Geometry check sheet. Reference: the model listing, model coordinates, mm. Face numbers are marked on the shaded views. A direction names the side the tool comes from. Give positions to 0.01 mm unless a question says otherwise; leave off trailing zeros. Write each loop counter-clockwise with the first axis right and the second up, starting at its lowest first coordinate (ties: lowest second). Pieces come first, ordered by that corner, then holes. Notation, with made-up numbers: (85.5, -34) -> (108.5, -34) arc R8 ccw to (108.5, -27) -> close; hole circle Ø1 at (35.25, 31.5). An arc over 180 degrees is marked (long way). Write item = value, one per line. Start each with the question number.
1. Set-up check for the marked faces 1 and 2: record each of +Z, -Z, +X, -X, +Y, -Y from which the full face is reachable in a straight line by a thin tool's end or side.
2. Thickness scan on line 1 along Y through (x, z) = (9.5, 4). Record the ranges inside material, lowest first.
3. Depth check by flat-ended pin: P1, Ø9.5, axis at y = 8.5, z = 12, coming from the +X side; P2, Ø12, axis at x = 12, y = 11, coming from the +Z side; P3, Ø10, axis at x = 5.5, y = 9, coming from the +Z side. Enter the tip coordinate at first touch or a pass-through.
4. Cross-section at A-A, the plane y = 7.25. Record the cut outline in (x, z).
```python
from build123d import *

# Parameters (mm, degrees)
F1_DEPTH     = 20
F3_DEPTH     = 20
F4_R         = 3
F5_T1_DEPTH  = 16
F5_T3_DEPTH  = 16
F5_T5_DEPTH  = 3
F5_T7_DEPTH  = 3
F5_T9_DEPTH  = 3
F5_T11_DEPTH = 16
F5_S15_W     = 1
F5_S15_H     = 1
F5_T16_DEPTH = 1
F5_S21_W     = 1
F5_S21_H     = 1
F5_T22_DEPTH = 1
F5_S27_W     = 1
F5_S27_H     = 1
F5_T28_DEPTH = 1
F5_T32_ANGLE = 90
F5_T34_ANGLE = 90
F5_T36_ANGLE = 90


# Not quite as in the source:
# - a fillet or chamfer that OpenCascade refuses, or shapes differently, is made with other operations: its cross-section is extruded or revolved along the edge and cut away or added


with BuildPart() as f1:
    # F0 (on Top) → F1 (new body)
    with BuildSketch(Plane.XY):
        Polygon((0, 20), (0, 0), (20, 0), (20, 1.5), (1.5, 1.5), (1.5, 20), align=None)
    extrude(amount=F1_DEPTH)

    # F2 (on Front) → F3 (join)
    with BuildSketch(Plane.XZ):
        Polygon((0, 20), (0, 0), (20, 0), (20, 1.5), (1.5, 1.5), (1.5, 20), align=None)
    extrude(amount=-F3_DEPTH)

    # F4
    f4_edges = [f1.edges().sort_by_distance(p)[0] for p in [
        (0, 0, 10),
        (0, 10, 0),
        (10, 0, 0),
    ]]
    fillet(f4_edges, radius=F4_R)

    # F5: fillet of radius 1 on 12 edges, made by hand

    # F5_s2 → F5_t1 (cut)
    with BuildSketch(Plane.XZ.offset(-19)):
        with BuildLine():
            ThreePointArc((0, 19), (0.2928932188, 19.7071067812), (1, 20))
            Line((1, 20), (0, 20))
            Line((0, 20), (0, 19))
        make_face()
        with BuildLine():
            ThreePointArc((19, 0), (19.7071067812, 0.2928932188), (20, 1))
            Line((20, 1), (20, 0))
            Line((20, 0), (19, 0))
        make_face()
    extrude(amount=F5_T1_DEPTH, mode=Mode.SUBTRACT)

    # F5_s4 → F5_t3 (cut)
    with BuildSketch(Plane.YZ.offset(3)):
        with BuildLine():
            ThreePointArc((20, 1), (19.7071067812, 0.2928932188), (19, 0))
            Line((19, 0), (20, 0))
            Line((20, 0), (20, 1))
        make_face()
        with BuildLine():
            ThreePointArc((1, 20), (0.2928932188, 19.7071067812), (0, 19))
            Line((0, 19), (0, 20))
            Line((0, 20), (1, 20))
        make_face()
    extrude(amount=F5_T3_DEPTH, mode=Mode.SUBTRACT)

    # F5_s6 → F5_t5 (cut)
    with BuildSketch(Plane.YZ.offset(1)):
        with BuildLine():
            ThreePointArc((20, 19), (19.7071067812, 19.7071067812), (19, 20))
            Line((19, 20), (20, 20))
            Line((20, 20), (20, 19))
        make_face()
    extrude(amount=F5_T5_DEPTH, mode=Mode.SUBTRACT)

    # F5_s8 → F5_t7 (cut)
    with BuildSketch(Plane.XY.offset(1)):
        with BuildLine():
            ThreePointArc((19, 20), (19.7071067812, 19.7071067812), (20, 19))
            Line((20, 19), (20, 20))
            Line((20, 20), (19, 20))
        make_face()
    extrude(amount=F5_T7_DEPTH, mode=Mode.SUBTRACT)

    # F5_s10 → F5_t9 (cut)
    with BuildSketch(Plane.XZ.offset(-4)):
        with BuildLine():
            ThreePointArc((19, 20), (19.7071067812, 19.7071067812), (20, 19))
            Line((20, 19), (20, 20))
            Line((20, 20), (19, 20))
        make_face()
    extrude(amount=F5_T9_DEPTH, mode=Mode.SUBTRACT)

    # F5_s12 → F5_t11 (cut)
    with BuildSketch(Plane.XY.offset(3)):
        with BuildLine():
            ThreePointArc((0, 19), (0.2928932188, 19.7071067812), (1, 20))
            Line((1, 20), (0, 20))
            Line((0, 20), (0, 19))
        make_face()
        with BuildLine():
            ThreePointArc((20, 1), (19.7071067812, 0.2928932188), (19, 0))
            Line((19, 0), (20, 0))
            Line((20, 0), (20, 1))
        make_face()
    extrude(amount=F5_T11_DEPTH, mode=Mode.SUBTRACT)


with BuildPart() as f5_tool14:
    # F5_s15 → F5_t16 (new body)
    with BuildSketch(Plane.YZ.offset(1)):
        with Locations((19.5, 19.5)):
            Rectangle(F5_S15_W, F5_S15_H)
    extrude(amount=-F5_T16_DEPTH)

    # F5_s17 → F5_t18 (revolve, cut)
    with BuildSketch(Plane(origin=(1, 19, 19), x_dir=(0, -0.7071067812, -0.7071067812), z_dir=(0, 0.7071067812, -0.7071067812))):
        with BuildLine():
            ThreePointArc((0, -1), (1, 0), (0, 1))
            Line((0, 1), (0, -1))
        make_face()
    revolve(axis=Axis((1, 19, 19), (-1, 0, 0)), mode=Mode.SUBTRACT)


with BuildPart() as f1_1:
    add(f1.part)

    # F5_t13: cut F5_tool14
    add(f5_tool14.part, mode=Mode.SUBTRACT)


with BuildPart() as f5_tool20:
    # F5_s21 → F5_t22 (new body)
    with BuildSketch(Plane.XZ.offset(-19)):
        with Locations((19.5, 0.5)):
            Rectangle(F5_S21_W, F5_S21_H)
    extrude(amount=-F5_T22_DEPTH)

    # F5_s23 → F5_t24 (revolve, cut)
    with BuildSketch(Plane(origin=(19, 19, 1), x_dir=(-0.7071067812, 0, 0.7071067812), z_dir=(-0.7071067812, 0, -0.7071067812))):
        with BuildLine():
            ThreePointArc((0, -1), (1, 0), (0, 1))
            Line((0, 1), (0, -1))
        make_face()
    revolve(axis=Axis((19, 19, 1), (0, 1, 0)), mode=Mode.SUBTRACT)


with BuildPart() as f1_2:
    add(f1_1.part)

    # F5_t19: cut F5_tool20
    add(f5_tool20.part, mode=Mode.SUBTRACT)


with BuildPart() as f5_tool26:
    # F5_s27 → F5_t28 (new body)
    with BuildSketch(Plane.XZ.offset(-1)):
        with Locations((19.5, 19.5)):
            Rectangle(F5_S27_W, F5_S27_H)
    extrude(amount=F5_T28_DEPTH)

    # F5_s29 → F5_t30 (revolve, cut)
    with BuildSketch(Plane(origin=(19, 1, 19), x_dir=(-0.7071067812, 0, -0.7071067812), z_dir=(-0.7071067812, 0, 0.7071067812))):
        with BuildLine():
            ThreePointArc((0, -1), (1, 0), (0, 1))
            Line((0, 1), (0, -1))
        make_face()
    revolve(axis=Axis((19, 1, 19), (0, -1, 0)), mode=Mode.SUBTRACT)


with BuildPart() as f1_3:
    add(f1_2.part)

    # F5_t25: cut F5_tool26
    add(f5_tool26.part, mode=Mode.SUBTRACT)

    # F5_s31 → F5_t32 (revolve, cut)
    with BuildSketch(Plane.XY.offset(3)):
        with BuildLine():
            ThreePointArc((1, 20), (0.2928932188, 19.7071067812), (0, 19))
            Line((0, 19), (0, 20))
            Line((0, 20), (1, 20))
        make_face()
    revolve(axis=Axis((3, 20, 3), (0, -1, 0)), revolution_arc=F5_T32_ANGLE, mode=Mode.SUBTRACT)

    # F5_s33 → F5_t34 (revolve, cut)
    with BuildSketch(Plane.XZ.offset(-3)):
        with BuildLine():
            ThreePointArc((1, 20), (0.2928932188, 19.7071067812), (0, 19))
            Line((0, 19), (0, 20))
            Line((0, 20), (1, 20))
        make_face()
    revolve(axis=Axis((3, 3, 20), (0, 0, 1)), revolution_arc=F5_T34_ANGLE, mode=Mode.SUBTRACT)

    # F5_s35 → F5_t36 (revolve, cut)
    with BuildSketch(Plane.XZ.offset(-3)):
        with BuildLine():
            ThreePointArc((20, 1), (19.7071067812, 0.2928932188), (19, 0))
            Line((19, 0), (20, 0))
            Line((20, 0), (20, 1))
        make_face()
    revolve(axis=Axis((20, 3, 3), (-1, 0, 0)), revolution_arc=F5_T36_ANGLE, mode=Mode.SUBTRACT)


solid = f1_3.part
```
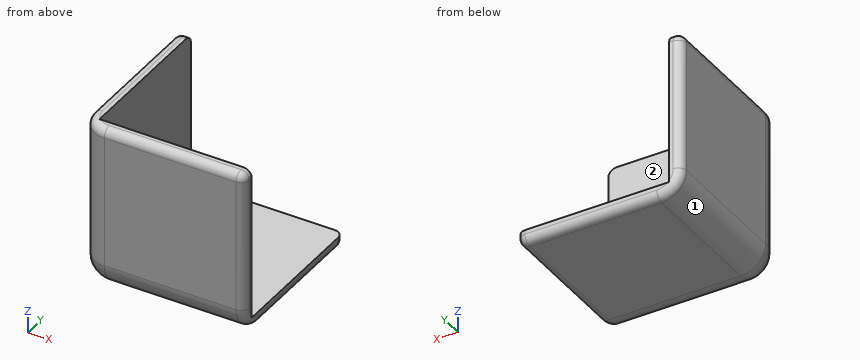
Answers:
q1.face_1 = -Z, -X, +Y, -Y
q1.face_2 = +Z, +X, +Y
q2.line_1 = 0 to 1.5
q3.P1 = 1.5
q3.P2 = 1.5
q3.P3 = 20
q4.outline = (0, 3) arc R3 ccw to (3, 0) -> (19, 0) arc R1 ccw to (20, 1) -> (20, 1.5) -> (1.5, 1.5) -> (1.5, 20) -> (1, 20) arc R1 ccw to (0, 19) -> close
